Work out the finished part from the listing and answer in its coordinate system (mm). Face numbers are marked on the shaded views. Coordinates: 2 decimals unless noted, no trailing zeros. Order: outer loops, then holes, each group sorted by start corner. A loop starts at its lowest first (then second) coordinate and runs counter-clockwise, first axis right, second up. Notation, with made-up numbers: M 45,45 L 81,45 A18 cw 81,64 Z; hole C 7,24 d9. An arc over 180 degrees is marked long. Answer in a Markdown table with one row per item. Add a question column.
Item 1: The mould has two halves that part along X. Classify the marked faces 1 and 2: released by +X, released by -X, zero draft, split by the parting line, or undercut.
Item 2: Flat-ended cylindrical pins translate along their axes: pin 1 Ø1.8 at (x, z) = (19.5, 1.5) entering from -Y; pin 2 Ø1 at (y, z) = (17, 5) entering from +X. Find the tip coordinate at first contact, or state that the pin passes through.
Item 3: The part is cut by section A-A (y = -14.5). Write down the section's boundary in (x, z), then the cut area to 3 significant figures.
Item 4: The part is cut by section B-B (z = 3.5). State how many separate pieces and enclosed holes the cut face has, then the cut area to 3 significant figures.
Item 5: Consider line 1 (Y direction, x = 6.35, z = 2.25); line 2 (X direction, y = -25.5, z = 3); line 3 (Y direction, x = -18.5, z = 5.75). Determine where each line is inside the solid, lowest interval first. Write a range as from..to.
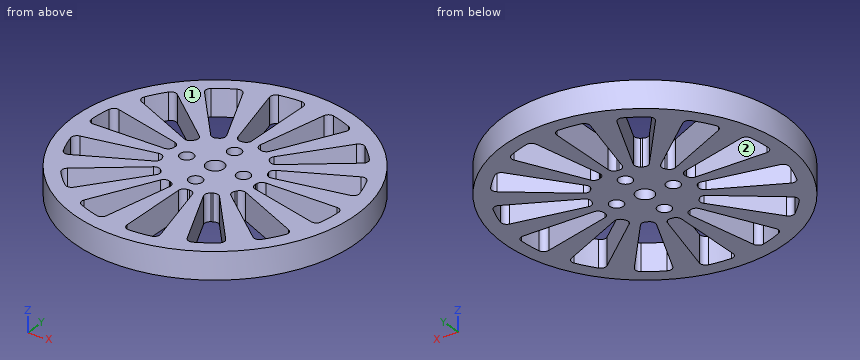
from build123d import *

# Parameters (mm, degrees)
SKETCH1_R           = 31.75
SKETCH1_R_2         = 1.524
SKETCH1_R_3         = 2
BOSS_EXTRUDE1_DEPTH = 6.096
CUT_EXTRUDE1_REACH  = 47.313
CIRPATTERN1_COUNT   = 14


with BuildPart() as part:
    # Sketch1 → Boss-Extrude1 (new body)
    with BuildSketch(Plane.XY):
        with Locations(Location((0, 0, 0), (0, 0, 180))):
            Circle(SKETCH1_R)
        with Locations(Location((0, 6.35, 0), (0, 0, 180))):
            Circle(SKETCH1_R_2, mode=Mode.SUBTRACT)
        with Locations(Location((6.35, 0, 0), (0, 0, 180))):
            Circle(SKETCH1_R_2, mode=Mode.SUBTRACT)
        with Locations(Location((0, -6.35, 0), (0, 0, 180))):
            Circle(SKETCH1_R_2, mode=Mode.SUBTRACT)
        with Locations(Location((-6.35, 0, 0), (0, 0, 180))):
            Circle(SKETCH1_R_2, mode=Mode.SUBTRACT)
        with Locations(Location((0, 0, 0), (0, 0, 180))):
            Circle(SKETCH1_R_3, mode=Mode.SUBTRACT)
    extrude(amount=BOSS_EXTRUDE1_DEPTH)

    # Sketch2 → Cut-Extrude1 (cut, up to next)
    with BuildSketch(Plane.XY.offset(6.096), mode=Mode.PRIVATE) as cut_extrude1_sk1:
        with BuildLine():
            Line((-27.275449126, 0), (-11.359225326, 0))
            ThreePointArc((-11.359225326, 0), (-10.512558659, 0.32339789), (-10.097089178, 1.128888889))
            ThreePointArc((-10.097089178, 1.128888889), (-10.073079792, 1.326146113), (-10.045217152, 1.522896047))
            ThreePointArc((-10.045217152, 1.522896047), (-10.238053442, 2.40847202), (-10.972169109, 2.939983852))
            Line((-10.972169109, 2.939983852), (-26.346060734, 7.059405697))
            ThreePointArc((-26.346060734, 7.059405697), (-27.335173973, 6.917463102), (-27.915447476, 6.103967335))
            ThreePointArc((-27.915447476, 6.103967335), (-28.330536914, 3.729785943), (-28.544074666, 1.329069767))
            ThreePointArc((-28.544074666, 1.329069767), (-28.194121702, 0.393107363), (-27.275449126, 0))
        make_face()
    cut_extrude1_tool1 = extrude(cut_extrude1_sk1.sketch, amount=-CUT_EXTRUDE1_REACH, mode=Mode.PRIVATE) & part.part
    cut_extrude1 = cut_extrude1_tool1.solids().sort_by_distance((-20.595833, 2.711493, 6.096))[0]
    add(cut_extrude1, mode=Mode.SUBTRACT)

    # CirPattern1: Cut-Extrude1 ×14 about axis
    cirpattern1_axis = Axis((0, 0, 0), (0, 0, 1))
    for i in range(1, CIRPATTERN1_COUNT):
        add(cut_extrude1.rotate(cirpattern1_axis, i * 360 / CIRPATTERN1_COUNT), mode=Mode.SUBTRACT)


solid = part.part
Reply:
| question | item | result |
|---|---|---|
| 1 | face 1 | zero draft |
| 1 | face 2 | undercut |
| 2 | pin 1 | stops at y = -25.73 |
| 2 | pin 2 | stops at x = 27.13 |
| 3 | outline | M -28.25,0 L -19.65,0 L -19.65,6.1 L -28.25,6.1 Z; M -11.56,0 L -7.66,0 L -7.66,6.1 L -11.56,6.1 Z; M -3.31,0 L -0.54,0 L -0.54,6.1 L -3.31,6.1 Z; M 3.31,0 L 6.33,0 L 6.33,6.1 L 3.31,6.1 Z; M 11.56,0 L 16.85,0 L 16.85,6.1 L 11.56,6.1 Z; M 24.62,0 L 28.25,0 L 28.25,6.1 L 24.62,6.1 Z |
| 3 | area | 166 mm2 |
| 4 | separate pieces | 1 |
| 4 | enclosed holes | 19 |
| 4 | area | 1,840 mm2 |
| 5 | line 1 | y = -31.11..-14.55, -8.43..-1.52, 1.52..12.01, 27.14..31.11 |
| 5 | line 2 | x = -18.92..-12.61, -5.82..-0.95, 5.82..11.3, 12.89..18.92 |
| 5 | line 3 | y = -25.8..-21.7, -13.65..-8.91, -3.5..0, 4.96..8.91, 15.92..25.8 |
